Could you check a few things on this model? Use its own coordinates, in mm. A direction names the side the tool comes from. Round coordinates to 2 decimals unless told otherwise and drop trailing zeros. Write each loop counter-clockwise with the first axis right and the second up, starting at its lowest first coordinate (ties: lowest second). Pieces come first, ordered by that corner, then holes. Notation, with made-up numbers: (47.5, -3) -> (63.5, -3) arc R38 ccw to (63.5, 36) -> close; hole circle Ø6 at (56.5, 41.25). An arc over 180 degrees is marked (long way). Return JSON: item names as keys, results as strings.
from build123d import *

# Parameters (mm, degrees)
F0_R     = 25.4
F1_DEPTH = 3.429


# Not quite as in the source:
# - ends of sketch curves that miss each other by under 0.0002 mm in the source are joined


with BuildPart() as f1:
    # F0 (on Front) → F1 (new body)
    with BuildSketch(Plane.XZ):
        with BuildLine():
            ThreePointArc((41.7896266471, 178.027378047), (41.789613947, 185.885114853), (49.647350753, 185.8851021529))
            Line((49.647350753, 185.8851021529), (80.9744634, 154.557984))
            ThreePointArc((80.9744634, 154.557984), (85.932800118, 201.4235329487), (45.972476, 226.4062528))
            Line((45.972476, 226.4062528), (6.888226, 226.4062528))
            Line((6.888226, 226.4062528), (6.888226, 229.5812528))
            Line((6.888226, 229.5812528), (-10.891774, 229.5812528))
            Line((-10.891774, 229.5812528), (-10.891774, 226.4062528))
            Line((-10.891774, 226.4062528), (-119.857774, 226.4062528))
            Line((-119.857774, 226.4062528), (-119.857774, 229.5812528))
            Line((-119.857774, 229.5812528), (-137.637774, 229.5812528))
            Line((-137.637774, 229.5812528), (-137.637774, 226.4062528))
            Line((-137.637774, 226.4062528), (-240.031524, 226.4062528))
            Line((-240.031524, 226.4062528), (-240.031524, 194.0212528))
            Line((-240.031524, 194.0212528), (-243.206524, 194.0212528))
            Line((-243.206524, 194.0212528), (-243.206524, 176.2412528))
            Line((-243.206524, 176.2412528), (-240.031524, 176.2412528))
            Line((-240.031524, 176.2412528), (-240.031524, 143.8562528))
            Line((-240.031524, 143.8562528), (-163.323524, 142.1719534))
            Line((-163.323524, 142.1719534), (-163.323524, 138.7199156))
            Line((-163.323524, 138.7199156), (-145.543524, 138.7199156))
            Line((-145.543524, 138.7199156), (-145.543524, 141.7815554))
            Line((-145.543524, 141.7815554), (-36.2456222, 139.3816618))
            Line((-36.2456222, 139.3816618), (-36.3153198, 136.2074238))
            Line((-36.3153198, 136.2074238), (-18.5353198, 135.8170258))
            Line((-18.5353198, 135.8170258), (-18.4656222, 138.9912638))
            Line((-18.4656222, 138.9912638), (47.67707, 137.5389426))
            ThreePointArc((47.67707, 137.5389426), (61.0963656021, 140.1582808001), (73.0847311317, 146.7322819609))
            Line((73.0847311317, 146.7322819609), (41.7896266471, 178.027378047))
        make_face()
        with Locations((-195.7019962, 185.2907394)):
            Circle(F0_R, mode=Mode.SUBTRACT)
        with Locations((-131.8551084, 185.2907394)):
            Circle(F0_R, mode=Mode.SUBTRACT)
        with Locations((-68.6405282, 185.2907394)):
            Circle(F0_R, mode=Mode.SUBTRACT)
        with Locations((-5.0234596, 185.2907394)):
            Circle(F0_R, mode=Mode.SUBTRACT)
    extrude(amount=F1_DEPTH)


solid = f1.part
1) I want a section at C-C, the plane z = 201.5. Please give me the cut outline in (x, y), and give its area (3 significant figures).
Return value:
{"outline": "(-240.03, -3.43) -> (-215.26, -3.43) -> (-215.26, 0) -> (-240.03, 0) -> close; (-176.15, -3.43) -> (-151.41, -3.43) -> (-151.41, 0) -> (-176.15, 0) -> close; (-112.3, -3.43) -> (-88.2, -3.43) -> (-88.2, 0) -> (-112.3, 0) -> close; (-49.08, -3.43) -> (-24.58, -3.43) -> (-24.58, 0) -> (-49.08, 0) -> close; (14.53, -3.43) -> (85.9, -3.43) -> (85.9, 0) -> (14.53, 0) -> close", "area": "581 mm²"}
2) For faces 4 (the face through (57.656, -1.69, 162.161)), 5 (the face through (86.23, -1.69, 200.8)), which set-ups out of +Z, -Z, +X, -X, +Y, -Y let a thin tool reach every point of the face, with its end or its side?
Return value:
{"face 4": "+Y, -Y", "face 5": "+X, +Y, -Y"}
3) I want a section at D-D, the plane y = -1.95. Count the separate pieces of the cut face and the enclosed holes in it, and give its area (3 significant figures).
Return value:
{"separate pieces": "1", "enclosed holes": "4", "area": "19,200 mm²"}
4) Will these pins go through, and if not, where does the flat tip stop? pin 1 Ø1 at (x, y) = (20.5, -2.5) entering from +Z; pin 2 Ø1.6 at (y, z) = (-1, 228.5) entering from -X; pin 3 Ø1.5 at (y, z) = (-2, 163) entering from +X.
Return value:
{"pin 1": "z = 226.41", "pin 2": "x = -137.64", "pin 3": "x = 86.52"}
5) If I drill on probe 1 along X at (y, z) = (-2.5, 163.5); probe 2 along X at (y, z) = (-1.4, 193.5); probe 3 along X at (y, z) = (-1.35, 198), over which ranges is the centre line in solid material (lowest first)? Write a range as [from, to].
Return value:
{"probe 1": "[-240.03, -208.75], [-182.65, -144.91], [-118.8, -81.69], [-55.59, -18.07], [8.03, 56.32], [72.03, 86.41]", "probe 2": "[-243.21, -219.74], [-171.67, -155.89], [-107.82, -92.68], [-44.6, -29.06], [19.01, 88.9]", "probe 3": "[-240.03, -217.69], [-173.71, -153.85], [-109.86, -90.63], [-46.65, -27.02], [16.97, 87.43]"}
6) I want a section at B-B, the plane x = -176. Please give me the cut outline in (y, z), and give its area (3 significant figures).
Return value:
{"outline": "(-3.43, 142.45) -> (0, 142.45) -> (0, 169.26) -> (-3.43, 169.26) -> close; (-3.43, 201.32) -> (0, 201.32) -> (0, 226.41) -> (-3.43, 226.41) -> close", "area": "178 mm²"}
7) I want a section at A-A, the plane z = 172.5. Please give me the cut outline in (x, y), and give its area (3 significant figures).
Return value:
{"outline": "(-240.03, -3.43) -> (-217.65, -3.43) -> (-217.65, 0) -> (-240.03, 0) -> close; (-173.76, -3.43) -> (-153.8, -3.43) -> (-153.8, 0) -> (-173.76, 0) -> close; (-109.91, -3.43) -> (-90.58, -3.43) -> (-90.58, 0) -> (-109.91, 0) -> close; (-46.7, -3.43) -> (-26.97, -3.43) -> (-26.97, 0) -> (-46.7, 0) -> close; (16.92, -3.43) -> (47.32, -3.43) -> (47.32, 0) -> (16.92, 0) -> close; (63.03, -3.43) -> (89.4, -3.43) -> (89.4, 0) -> (63.03, 0) -> close", "area": "474 mm²"}
8) Thinking about a two-plate mould opening in Z: for faces 1 (the face through (60.916, -1.69, 140.093)), 2 (the face through (-79, -3.429, 215)), 3 (the face through (65.09, -1.69, 170.44)), which applies, pulls with the +Z half, pulls with the -Z half, needs draft (parallel to the pull), parting line crosses it, or undercut?
Return value:
{"face 1": "pulls with the -Z half", "face 2": "needs draft", "face 3": "undercut"}
